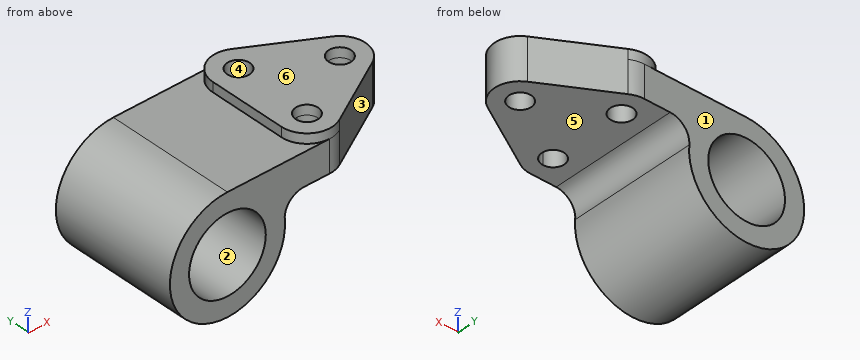
```python
from build123d import *

# Parameters (mm, degrees)
F0_R     = 19.05
F1_DEPTH = 63.5
F2_R     = 5.5626
F3_DEPTH = 4.7752
F6_DEPTH = 15.875
F7_R     = 5.5626
F8_DEPTH = 57.151


with BuildPart() as f1:
    # F0 (on Front) → F1 (new body)
    with BuildSketch(Plane.XZ):
        with BuildLine():
            Line((37.967478, 12.7), (50.8, 12.7))
            Line((50.8, 12.7), (50.8, 28.575))
            Line((50.8, 28.575), (0, 28.575))
            ThreePointArc((0, 28.575), (-19.345366, -21.030631), (28.475608, 2.38125))
            ThreePointArc((28.475608, 2.38125), (30.957268, 9.623455), (37.967478, 12.7))
        make_face()
        Circle(F0_R, mode=Mode.SUBTRACT)
    extrude(amount=F1_DEPTH)

    # F2 (on face) → F3 (join)
    with BuildSketch(Plane.XY.offset(28.575)):
        with BuildLine():
            ThreePointArc((57.36329, -1.827409), (44.557556, -1.640077), (38.1, -12.7))
            Line((38.1, -12.7), (38.1, -50.8))
            ThreePointArc((38.1, -50.8), (44.557556, -61.859923), (57.36329, -61.672591))
            Line((57.36329, -61.672591), (90.448286, -42.778332))
            ThreePointArc((90.448286, -42.778332), (96.8502, -31.75), (90.448286, -20.721668))
            Line((90.448286, -20.721668), (57.36329, -1.827409))
        make_face()
        with Locations((50.8, -50.8)):
            Circle(F2_R, mode=Mode.SUBTRACT)
        with Locations((50.8, -12.7)):
            Circle(F2_R, mode=Mode.SUBTRACT)
        with Locations((84.1502, -31.75)):
            Circle(F2_R, mode=Mode.SUBTRACT)
    extrude(amount=F3_DEPTH)

    # F5 (on face) + F4 (on face) → F6 (join)
    with BuildSketch(Plane(origin=(0, 0, 28.575), x_dir=(1, 0, 0), z_dir=(0, 0, -1))):
        with BuildLine():
            Line((90.448286, 42.778332), (57.36329, 61.672591))
            ThreePointArc((57.36329, 61.672591), (54.206472, 63.034621), (50.8, 63.5))
            Line((50.8, 63.5), (50.8, 56.3626))
            ThreePointArc((50.8, 56.3626), (56.3626, 50.8), (50.8, 45.2374))
            Line((50.8, 45.2374), (50.8, 18.2626))
            ThreePointArc((50.8, 18.2626), (56.3626, 12.7), (50.8, 7.1374))
            Line((50.8, 7.1374), (50.8, 0))
            ThreePointArc((50.8, 0), (54.206472, 0.465379), (57.36329, 1.827409))
            Line((57.36329, 1.827409), (90.448286, 20.721668))
            ThreePointArc((90.448286, 20.721668), (96.8502, 31.75), (90.448286, 42.778332))
        make_face()
    with BuildSketch(Plane(origin=(0, 0, 28.575), x_dir=(1, 0, 0), z_dir=(0, 0, -1))):
        with BuildLine():
            Line((90.448286, 42.778332), (57.36329, 61.672591))
            ThreePointArc((57.36329, 61.672591), (54.206472, 63.034621), (50.8, 63.5))
            Line((50.8, 63.5), (50.8, 56.3626))
            ThreePointArc((50.8, 56.3626), (56.3626, 50.8), (50.8, 45.2374))
            Line((50.8, 45.2374), (50.8, 18.2626))
            ThreePointArc((50.8, 18.2626), (56.3626, 12.7), (50.8, 7.1374))
            Line((50.8, 7.1374), (50.8, 0))
            ThreePointArc((50.8, 0), (54.206472, 0.465379), (57.36329, 1.827409))
            Line((57.36329, 1.827409), (90.448286, 20.721668))
            ThreePointArc((90.448286, 20.721668), (96.8502, 31.75), (90.448286, 42.778332))
        make_face()
    extrude(amount=F6_DEPTH)

    # F7 (on face) → F8 (cut, through all)
    with BuildSketch(Plane.XY.offset(28.575)):
        with Locations((50.8, -50.8)):
            Circle(F7_R)
        with Locations((50.8, -12.7)):
            Circle(F7_R)
        with Locations((84.1502, -31.75)):
            Circle(F7_R)
    extrude(amount=-F8_DEPTH, mode=Mode.SUBTRACT)


solid = f1.part
```
Check sheet for the modelled part. Datum: model origin and axes. Units: mm. Face numbers are marked on the shaded views. A direction names the side the tool comes from. Give positions to 0.01 mm unless a question says otherwise; leave off trailing zeros. Write each loop counter-clockwise with the first axis right and the second up, starting at its lowest first coordinate (ties: lowest second). Pieces come first, ordered by that corner, then holes.
Item 1: Scan lines: L1, parallel to Y at x = 50.8, z = 29; L2, parallel to Z at x = 0, y = -13 (3 decimals); L3, parallel to X at y = -51, z = 14. Record each from-to range of solid material in increasing order.
Item 2: Cross-section at D-D (x = -2). Enter the section's corners in (y, z).
Item 3: Cross-section at C-C (z = 17.5). Enter the section's corners in (x, y).
Item 4: Cross-section at B-B (y = -54). Enter the section's corners in (x, z) (3 decimals).
Item 5: Access from +Z, -Z, +X, -X, +Y, -Y to the whole of each face (thin tool, end or side, straight path). Record for the marked faces 5 and 6.
Item 6: Cross-section at A-A (z = 0). Enter the section's corners in (x, y) (3 decimals), and give its area (3 significant figures).
Item 7: Draft check along Y on the marked faces 1, 2, 3 and 4. Enter one of: released by +Y, released by -Y, zero draft, split by the parting line, or undercut.
Item 8: Gauge pin test, flat ends, axial feed: pin 1 (12 mm diameter, centred on y = -43, z = 12.5, fed in from +X); pin 2 (4 mm diameter, centred on x = 71.5, y = -51, fed in from -Z); pin 3 (1 mm diameter, centred on y = -39, z = -17.5, fed in from -X); pin 4 (6.5 mm diameter, centred on x = 50.8, y = -50.8, fed in from -Z). Record the tip position at first contact, or that the pin passes through.
Report:
1. L1: y = -63.5 to -56.36, -45.24 to -18.26, -7.14 to 0
1. L2: z = -28.575 to -19.05, 19.05 to 28.575
1. L3: x = -24.91 to -12.92, 12.92 to 45.24, 56.36 to 76.05
2. outline: (-63.5, -28.5) - (0, -28.5) - (0, -18.94) - (-63.5, -18.94) - close; (-63.5, 18.94) - (0, 18.94) - (0, 28.5) - (-63.5, 28.5) - close
3. outline: (-22.59, -63.5) - (-7.53, -63.5) - (-7.53, 0) - (-22.59, 0) - close; (7.53, -63.5) - (50.8, -63.5) arc R12.7 ccw to (57.36, -61.67) - (90.45, -42.78) arc R12.7 ccw to (90.45, -20.72) - (57.36, -1.83) arc R12.7 ccw to (50.8, 0) - (7.53, 0) - close; hole circle Ø11.13 at (50.8, -50.8); hole circle Ø11.13 at (50.8, -12.7); hole circle Ø11.13 at (84.15, -31.75)
4. outline: (0, 28.575) arc R28.575 ccw (long way) to (28.476, 2.381) arc R9.525 cw to (37.967, 12.7) - (46.25, 12.7) - (46.25, 33.35) - (38.51, 33.35) - (38.51, 28.575) - close; (55.35, 12.7) - (70.798, 12.7) - (70.798, 33.35) - (55.35, 33.35) - close; hole circle Ø38.1 at (0, 0)
5. face 5: -Z, +X, +Y, -Y
5. face 6: +Z, +X, -X, +Y, -Y
6. outline: (-28.575, -63.5) - (-19.05, -63.5) - (-19.05, 0) - (-28.575, 0) - close; (19.05, -63.5) - (28.575, -63.5) - (28.575, 0) - (19.05, 0) - close
6. area: 1,210 mm2
7. face 1: released by +Y
7. face 2: zero draft
7. face 3: released by -Y
7. face 4: undercut
8. pin 1: stops at x = 95.71
8. pin 2: stops at z = 12.7
8. pin 3: stops at x = -22.97
8. pin 4: passes through
